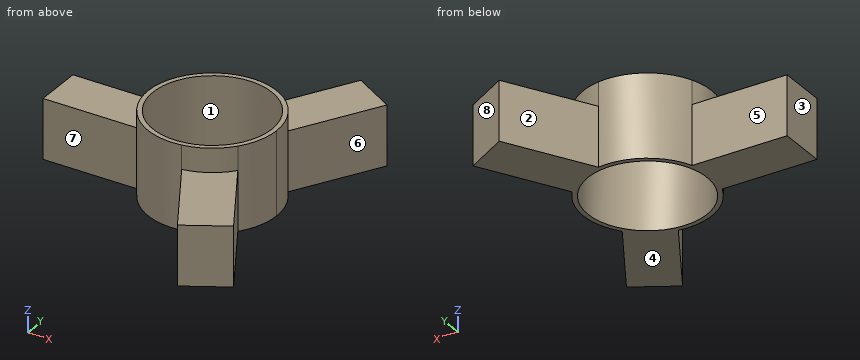
```python
from build123d import *

# Parameters (mm, degrees)
F0_R     = 25
F1_DEPTH = 35
F2_DEPTH = 25


with BuildPart() as f1:
    # F0 (on Top) → F1 (new body)
    with BuildSketch(Plane.XY):
        with BuildLine():
            ThreePointArc((21.20019, -16.719807), (25.508872, -8.848584), (27, 0))
            ThreePointArc((27, 0), (25.508872, 8.848584), (21.20019, 16.719807))
            ThreePointArc((21.20019, 16.719807), (13.5, 23.382686), (3.879682, 26.719807))
            ThreePointArc((3.879682, 26.719807), (-13.5, 23.382686), (-25.079872, 10))
            ThreePointArc((-25.079872, 10), (-27, 0), (-25.079872, -10))
            ThreePointArc((-25.079872, -10), (-13.5, -23.382686), (3.879682, -26.719807))
            ThreePointArc((3.879682, -26.719807), (13.5, -23.382686), (21.20019, -16.719807))
        make_face()
        Circle(F0_R, mode=Mode.SUBTRACT)
    extrude(amount=F1_DEPTH)

    # F0 (on Top) → F2 (join)
    with BuildSketch(Plane.XY):
        with BuildLine():
            ThreePointArc((-25.079872, -10), (-27, 0), (-25.079872, 10))
            Line((-25.079872, 10), (-65, 10))
            Line((-65, 10), (-65, -10))
            Line((-65, -10), (-25.079872, -10))
        make_face()
        with BuildLine():
            Line((41.160254, -51.291651), (21.20019, -16.719807))
            ThreePointArc((21.20019, -16.719807), (13.5, -23.382686), (3.879682, -26.719807))
            Line((3.879682, -26.719807), (23.839746, -61.291651))
            Line((23.839746, -61.291651), (41.160254, -51.291651))
        make_face()
        with BuildLine():
            ThreePointArc((3.879682, 26.719807), (13.5, 23.382686), (21.20019, 16.719807))
            Line((21.20019, 16.719807), (41.160254, 51.291651))
            Line((41.160254, 51.291651), (23.839746, 61.291651))
            Line((23.839746, 61.291651), (3.879682, 26.719807))
        make_face()
    extrude(amount=F2_DEPTH)


solid = f1.part
```
Could you check a few things on this model? Use its own coordinates, in mm. Face numbers are marked on the shaded views. A direction names the side the tool comes from. Give positions to 0.01 mm unless a question says otherwise; leave off trailing zeros. Loops run counter-clockwise (first coordinate to the right, second up) from the corner with the lowest first, then second, coordinate; pieces in that order, holes last. Notation, with made-up numbers: (68.5, 87.5) -> (114.5, 87.5) arc R28 ccw to (114.5, 122.5) -> close; hole circle Ø3 at (51.5, -19). An arc over 180 degrees is marked (long way). Put each result on its own line as item: value.
(1) Imagine slicing it at A-A on x = 0. Write out the boundary of the cut face in (y, z), plus the area to 3 significant figures.
Computed:
outline: (-27, 0) -> (-25, 0) -> (-25, 35) -> (-27, 35) -> close; (25, 0) -> (27, 0) -> (27, 35) -> (25, 35) -> close
area: 140 mm^2
(2) For the marked faces 4, 5, 6, 7 and 8, which set-ups out of +Z, -Z, +X, -X, +Y, -Y let a thin tool reach every point of the face, with its end or its side?
Computed:
face 4: -Z, +X, -X, +Y, -Y
face 5: +Z, -Z, -X, +Y
face 6: +Z, -Z, +X
face 7: +Z, -Z, -X, -Y
face 8: +Z, -Z, +X, +Y
(3) Imagine slicing it at B-B on z = 29.5. Write out the boundary of the cut face in (x, y).
Computed:
outline: (-25.08, -10) arc R27 ccw to (3.88, -26.72) arc R27 ccw to (21.2, -16.72) arc R27 ccw to (27, 0) arc R27 ccw to (21.2, 16.72) arc R27 ccw to (3.88, 26.72) arc R27 ccw to (-25.08, 10) arc R27 ccw to start; hole circle Ø50 at (0, 0)
(4) Please list where these lines run through material, in increasing order: probe 1 along Y at (x, z) = (0, 22); probe 2 along Z at (x, y) = (-42, 3); probe 3 along Y at (x, z) = (-39.5, 11.5). Write a range as [from, to].
Computed:
probe 1: [-27, -25], [25, 27]
probe 2: [0, 25]
probe 3: [-10, 10]
(5) Thinking about a two-plate mould opening in Y: for the marked faces 1, 2 and 3, which applies, pulls with the +Y half, pulls with the -Y half, needs draft (parallel to the pull), parting line crosses it, or undercut?
Computed:
face 1: undercut
face 2: pulls with the +Y half
face 3: needs draft
(6) Imagine slicing it at D-D on z = 17. Write out the boundary of the cut face in (x, y), plus the area to 3 significant figures.
Computed:
outline: (-65, -10) -> (-25.08, -10) arc R27 ccw to (3.88, -26.72) -> (23.84, -61.29) -> (41.16, -51.29) -> (21.2, -16.72) arc R27 ccw to (27, 0) arc R27 ccw to (21.2, 16.72) -> (41.16, 51.29) -> (23.84, 61.29) -> (3.88, 26.72) arc R27 ccw to (-25.08, 10) -> (-65, 10) -> close; hole circle Ø50 at (0, 0)
area: 2,640 mm^2
(7) Imagine slicing it at C-C on y = 14.5. Write out the boundary of the cut face in (x, z), plus the area to 3 significant figures.
Computed:
outline: (-22.78, 0) -> (-20.37, 0) -> (-20.37, 35) -> (-22.78, 35) -> close; (20.37, 0) -> (22.78, 0) -> (22.78, 35) -> (20.37, 35) -> close
area: 169 mm^2
(8) I'm going to push flat-ended pins straight in: pin 1 Ø4 at (x, z) = (-21, 20.5) entering from +Y; pin 2 Ø1 at (y, z) = (43.5, 13) entering from -X; pin 3 Ø1.5 at (x, z) = (7, 13.5) entering from +Y. Where does each tip first touch, or does it pass through?
Computed:
pin 1: y = 19.18
pin 2: x = 13.28
pin 3: y = 33.42
